from build123d import *

# Parameters (mm, degrees)
SKETCH1_R           = 0.8509
BOSS_EXTRUDE1_DEPTH = 3


with BuildPart() as part:
    # Sketch1 → Boss-Extrude1 (new body)
    with BuildSketch(Plane.XY):
        Polygon((15.691, 24.0041), (-15.691, 24.0041), (-15.691, 0), (-11.811, 0), (-11.811, 18.1091), (11.811, 18.1091), (11.811, 0), (15.691, 0), align=None)
        with Locations((-13.751, 12.0021)):
            Circle(SKETCH1_R, mode=Mode.SUBTRACT)
        with Locations(Location((13.751, 12.0021, 0), (0, 0, 180))):
            Circle(SKETCH1_R, mode=Mode.SUBTRACT)
    extrude(amount=BOSS_EXTRUDE1_DEPTH)


solid = part.part
Source: CAD feature listing. Evaluate the final solid. Frame: model axes, mm. A direction names the side the tool comes from. Coordinates: 2 decimals unless noted, no trailing zeros. Loops run counter-clockwise (first coordinate to the right, second up) from the corner with the lowest first, then second, coordinate; pieces in that order, holes last. Notation, with made-up numbers: M -6.5,28.25 L 19.5,28.25 A31 ccw 19.5,59.25 Z; hole C 5.25,50 d5. An arc over 180 degrees is marked long. Answer in a Markdown table with one row per item.
Q1. Section A-A on y = 3. Return the cut outline in (x, z), plus the area to 3 significant figures.
Answers below:
| item | result |
|---|---|
| outline | M -15.69,0 L -11.81,0 L -11.81,3 L -15.69,3 Z; M 11.81,0 L 15.69,0 L 15.69,3 L 11.81,3 Z |
| area | 23.3 mm^2 |
Q2. Ray query, probe 1 along X at (y, z) = (2.5, 0.4); probe 2 along X at (y, z) = (11.5, 2.05); probe 3 along Y at (x, z) = (8.5, 1.55). Return the intervals inside material, ascending. Write a range as from..to.
Answers below:
| item | result |
|---|---|
| probe 1 | x = -15.69..-11.81, 11.81..15.69 |
| probe 2 | x = -15.69..-14.44, -13.06..-11.81, 11.81..13.06, 14.44..15.69 |
| probe 3 | y = 18.11..24 |
Q3. Set-up query: faces 4 (the flat face through (11.811, 9, 1)), 5 (the flat face through (0, 24.004, 1)). Return all of +Z, -Z, +X, -X, +Y, -Y with unobstructed straight access to the full face (end or side cutting, diameter ignored); none if empty.
Answers below:
| item | result |
|---|---|
| face 4 | +Z, -Z, -Y |
| face 5 | +Z, -Z, +X, -X, +Y |
Q4. Draft query along X for faces 1 (the flat face through (15.691, 12, 1)), 2 (the flat face through (0, 20, 0)), 3 (the cylindrical face through (13.294, 11.285, 1.479)). Return one class per face: pulls with the +X half, pulls with the -X half, needs draft (parallel to the pull), parting line crosses it, or undercut.
Answers below:
| item | result |
|---|---|
| face 1 | pulls with the +X half |
| face 2 | needs draft |
| face 3 | undercut |
Q5. Section B-B on z = 0.6. Return the cut outline in (x, y).
Answers below:
| item | result |
|---|---|
| outline | M -15.69,0 L -11.81,0 L -11.81,18.11 L 11.81,18.11 L 11.81,0 L 15.69,0 L 15.69,24 L -15.69,24 Z; hole C -13.75,12 d1.7; hole C 13.75,12 d1.7 |
Q6. Section C-C on x = -9.5. Return the cut outline in (y, z), plus the area to 3 significant figures.
Answers below:
| item | result |
|---|---|
| outline | M 18.11,0 L 24,0 L 24,3 L 18.11,3 Z |
| area | 17.7 mm^2 |
Q7. First-contact query: pin 1 (1.5 mm diameter, centred on x = -6.5, z = 1, fed in from -Y). Flat tip, straight axial feed; report the tip coordinate or a pass-through.
Answers below:
| item | result |
|---|---|
| pin 1 | stops at y = 18.11 |
